The model under review builds one solid part; all positions refer to its coordinate system, in mm. Face numbers are marked on the shaded views. A direction names the side the tool comes from. Give positions to 0.01 mm unless a question says otherwise; leave off trailing zeros. Order: outer loops, then holes, each group sorted by start corner. A loop starts at its lowest first (then second) coordinate and runs counter-clockwise, first axis right, second up. Notation, with made-up numbers: (73.25, 57) - (122.25, 57) arc R34 cw to (122.25, 89) - close; hole circle Ø6 at (32.5, 64). An arc over 180 degrees is marked (long way). Write item = value, one per line. Start each with the question number.
1. For P1, Ø1, axis at x = -0.5, z = -3, coming from the -Y side; P2, Ø8, axis at x = 7.5, y = 17, coming from the +Z side; P3, Ø3, axis at x = -10, z = 13.5, coming from the -Y side; P4, Ø4, axis at y = 25, z = 10, coming from the -X side, all flat-tipped, find the tip position at first contact; note any pin that passes through.
2. We need section B-B, the plane x = -28. Give the boundary of the cut face in (y, z), and give its area (3 significant figures).
3. We need section C-C, the plane z = 4.5. Give the boundary of the cut face in (x, y).
4. We need section A-A, the plane y = 8.15. Give the boundary of the cut face in (x, z).
5. Wall thickness on probe 1 along Z at (x, y) = (-16, -25); probe 2 along Y at (x, z) = (8, -1.75); probe 3 along Y at (x, z) = (-10.5, 13.25): over which ranges is each line inside the solid? List them lowest first.
6. Mouldability with a two-part tool opening along Z and no side actions: class the marked faces 5, 6 and 7 as pulls with the +Z half, pulls with the -Z half, needs draft (parallel to the pull), parting line crosses it, or undercut.
7. We need section D-D, the plane y = -21. Give the boundary of the cut face in (x, z).
8. Machinability: for the marked faces 1, 2, 3 and 4, which of the approach directions +Z, -Z, +X, -X, +Y, -Y give a long, thin tool a straight path to every point of the face, cutting with its end or side? Answer none if there is none.
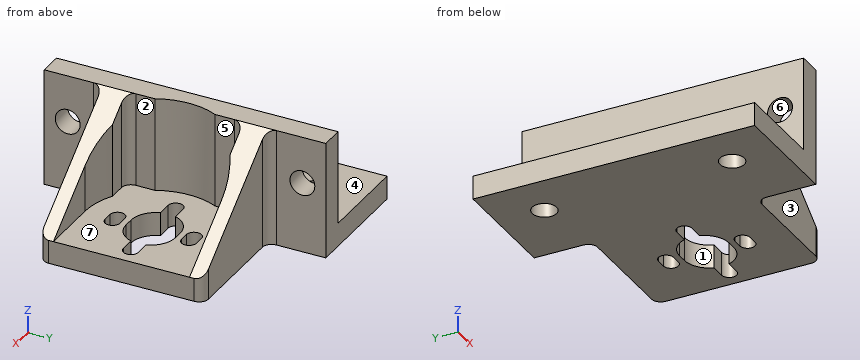
from build123d import *

# Parameters (mm, degrees)
SKETCH_R          = 2.6
PAD_DEPTH         = 20
PAD_DEPTH_BACK    = 5
SKETCH002_W       = 33.294622
SKETCH002_H       = 24.26609
POCKET001_DEPTH   = 12.5
SKETCH003_R       = 2.65
POCKET002_DEPTH   = 38.001
POCKET003_DEPTH   = 20.001
SKETCH001_W       = 20
SKETCH001_H       = 20
POCKET_DEPTH      = 30.001
POCKET_DEPTH_BACK = -30.001
FILLET_R          = 2


with BuildPart() as part:
    # Sketch → Pad (new body, two sides)
    with BuildSketch(Plane.XY) as pad_sk:
        Polygon((-13, 17.5), (13, 17.5), (13, -17.5), (-13, -17.5), (-13, -30), (-38, -30), (-38, 30), (-13, 30), align=None)
        with Locations((-28, 20)):
            Circle(SKETCH_R, mode=Mode.SUBTRACT)
        with Locations((-28, -20)):
            Circle(SKETCH_R, mode=Mode.SUBTRACT)
        with BuildLine():
            Line((-1, -5.25), (1, -5.25))
            ThreePointArc((1, -5.25), (4.095359, -4.24043), (6.00025, -1.6))
            Line((6.00025, -1.6), (9.15, -1.6))
            ThreePointArc((9.15, -1.6), (10.75, 0), (9.15, 1.6))
            Line((6.00025, 1.6), (9.15, 1.6))
            ThreePointArc((6.00025, 1.6), (4.095359, 4.24043), (1, 5.25))
            Line((-1, 5.25), (1, 5.25))
            ThreePointArc((-1, 5.25), (-4.095359, 4.24043), (-6.00025, 1.6))
            Line((-9.15, 1.6), (-6.00025, 1.6))
            ThreePointArc((-9.15, 1.6), (-10.75, 0), (-9.15, -1.6))
            Line((-9.15, -1.6), (-6.00025, -1.6))
            ThreePointArc((-6.00025, -1.6), (-4.095359, -4.24043), (-1, -5.25))
        make_face(mode=Mode.SUBTRACT)
        with BuildLine():
            ThreePointArc((-1, 9.75), (-2.6, 8.15), (-1, 6.55))
            Line((-1, 6.55), (1, 6.55))
            ThreePointArc((1, 6.55), (2.6, 8.15), (1, 9.75))
            Line((-1, 9.75), (1, 9.75))
        make_face(mode=Mode.SUBTRACT)
        with BuildLine():
            ThreePointArc((-1, -6.55), (-2.6, -8.15), (-1, -9.75))
            Line((-1, -9.75), (1, -9.75))
            ThreePointArc((1, -9.75), (2.6, -8.15), (1, -6.55))
            Line((-1, -6.55), (1, -6.55))
        make_face(mode=Mode.SUBTRACT)
    extrude(amount=PAD_DEPTH)
    extrude(pad_sk.sketch, amount=-PAD_DEPTH_BACK)

    # Sketch002 → Pocket001 (cut, symmetric)
    with BuildSketch(Plane.XZ):
        with Locations((3.647311, 12.133045)):
            Rectangle(SKETCH002_W, SKETCH002_H)
    extrude(amount=POCKET001_DEPTH, both=True, mode=Mode.SUBTRACT)

    # Sketch003 → Pocket002 (cut, through all)
    with BuildSketch(Plane.YZ):
        with Locations((-25, 10)):
            Circle(SKETCH003_R)
        with Locations((25, 10)):
            Circle(SKETCH003_R)
    extrude(amount=-POCKET002_DEPTH, mode=Mode.SUBTRACT)

    # Sketch004 → Pocket003 (cut, through all)
    with BuildSketch(Plane.XY):
        with BuildLine():
            ThreePointArc((0, 14.5), (-14.5, 0), (0, -14.5))
            Line((29.411848, -14.5), (0, -14.5))
            Line((29.411848, 14.5), (29.411848, -14.5))
            Line((0, 14.5), (29.411848, 14.5))
        make_face()
    extrude(amount=POCKET003_DEPTH, mode=Mode.SUBTRACT)

    # Sketch001 → Pocket (cut, two sides)
    with BuildSketch(Plane.XZ) as pocket_sk:
        with Locations((-28, 10)):
            Rectangle(SKETCH001_W, SKETCH001_H)
        Polygon((-13, 20), (13, 20), (13, 0), align=None)
    extrude(amount=-POCKET_DEPTH, mode=Mode.SUBTRACT)
    extrude(pocket_sk.sketch, amount=-POCKET_DEPTH_BACK, mode=Mode.SUBTRACT)

    # Fillet
    fillet_edges = [part.edges().sort_by_distance(p)[0] for p in [
        (-13, -17.5, 7.5),
        (13, -17.5, -2.5),
        (13, 17.5, -2.5),
        (-13, 17.5, 7.5),
        (-13, 12.5, 10),
        (-13, -12.5, 10),
    ]]
    fillet(fillet_edges, radius=FILLET_R)


solid = part.part
Model answer:
q1.P1 = -17.5
q1.P2 = 7.31
q1.P3 = -17.56
q1.P4 = through
q2.outline = (-30, -5) - (-22.6, -5) - (-22.6, 0) - (-30, 0) - close; (-17.4, -5) - (17.4, -5) - (17.4, 0) - (-17.4, 0) - close; (22.6, -5) - (30, -5) - (30, 0) - (22.6, 0) - close
q2.area = 248 mm2
q3.outline = (-18, -30) - (-13, -30) - (-13, -19.5) arc R2 cw to (-11, -17.5) - (7.15, -17.5) - (7.15, -14.5) - (0, -14.5) arc R14.5 cw to (-7.35, -12.5) - (-11, -12.5) arc R2 cw to (-13, -10.5) - (-13, -6.42) arc R14.5 cw to (-13, 6.42) - (-13, 10.5) arc R2 cw to (-11, 12.5) - (-7.35, 12.5) arc R14.5 cw to (0, 14.5) - (7.15, 14.5) - (7.15, 17.5) - (-11, 17.5) arc R2 cw to (-13, 19.5) - (-13, 30) - (-18, 30) - close
q4.outline = (-38, -5) - (-2.6, -5) - (-2.6, 0) - (-13, 0) - (-13, 20) - (-18, 20) - (-18, 0) - (-38, 0) - close; (2.6, -5) - (13, -5) - (13, 0) - (2.6, 0) - close
q5.probe_1 = -5 to 7.35, 12.65 to 20
q5.probe_2 = -17.5 to -1.6, 1.6 to 17.5
q5.probe_3 = -17.5 to -12.5, 12.5 to 17.5
q6.face_5 = needs draft
q6.face_6 = undercut
q6.face_7 = pulls with the +Z half
q7.outline = (-38, -5) - (-30.4, -5) - (-30.4, 0) - (-38, 0) - close; (-25.6, -5) - (-13, -5) - (-13, 20) - (-18, 20) - (-18, 0) - (-25.6, 0) - close
q8.face_1 = +Z, -Z
q8.face_2 = +Z, +X
q8.face_3 = +Z, -Z, +X, -Y
q8.face_4 = +Z, -X, +Y, -Y
